For this review, take the finished solid that the model builds, in its own axes (mm). A direction names the side the tool comes from. Give positions to 0.01 mm unless a question says otherwise; leave off trailing zeros. Loops run counter-clockwise (first coordinate to the right, second up) from the corner with the lowest first, then second, coordinate; pieces in that order, holes last. Notation, with made-up numbers: (-30.75, 88) - (22.25, 88) arc R15 cw to (22.25, 116) - close; hole circle Ø2 at (83, -16). An arc over 180 degrees is marked (long way). Put each result on its own line as item: value.
Autodesk Inventor part; units mm, degrees
ref_plane "YZ Plane" through (0, 0, 0) normal (1, 0, 0) x (0, 1, 0)
ref_plane "XZ Plane" through (0, 0, 0) normal (0, 1, 0) x (-1, 0, 0)
ref_plane "XY Plane" through (0, 0, 0) normal (0, 0, 1) x (1, 0, 0)
sketch "Sketch1" plane through (0, 0, 0) normal (0, 1, 0) x (-1, 0, 0)
  line L0 (0, 0) -> (-139.7, 0)
  line L1 (-139.7, 0) -> (-139.7, -139.7)
  line L2 (-139.7, -139.7) -> (0, -139.7)
  line L3 (0, -139.7) -> (0, 0)
  dimension "d0" = 139.7
  dimension "d1" = 139.7
extrude "Extrusion1" add sketch "Sketch1" along normal blind 25.4
sketch "Sketch2" plane through (0, 25.4, 0) normal (0, 1, 0) x (1, 0, 0)
  circle A0 centre (104.775, 34.925) radius 25.4
  line L0 (0, 0) -> (139.7, 0)
  line L1 (139.7, 0) -> (139.7, 139.7)
  line L2 (139.7, 139.7) -> (0, 139.7)
  line L3 (0, 139.7) -> (0, 0)
  dimension "d4" = 50.8
  dimension "d5" = 34.925
  dimension "d6" = 34.925
extrude "Extrusion2" cut sketch "Sketch2" against normal blind 3.175 contours A0
sketch "Sketch3" plane through (104.775, 22.225, -34.925) normal (0, 1, 0) x (1, 0, 0)
  circle A0 centre (0, 0) radius 19.05
  point P0 (-104.775, -34.925)
  dimension "d9" = 38.1
extrude "Extrusion3" cut sketch "Sketch3" against normal blind 3.937
equation "\"d5\" = d6"
properties part number "Saber plaque"
1) Draft analysis for pull direction X (two halves, no side actions). For faces 1 (the face through (139.7, 13, -69)), 2 (the face through (108, 22.225, -54)), 3 (the face through (101.47, 23.83, -60.11)), 4 (the face through (71, 13, -139.7)), state which applies: pulls with the +X half, pulls with the -X half, needs draft (parallel to the pull), parting line crosses it, or undercut.
Geometry check:
face 1: pulls with the +X half
face 2: undercut
face 3: undercut
face 4: needs draft
2) Take a section at A-A on x = 98.5. State the section outline as (y, z) points (3 decimals), and give its area (3 significant figures).
Geometry check:
outline: (0, -139.7) - (25.4, -139.7) - (25.4, -59.538) - (22.225, -59.538) - (22.225, -52.912) - (18.288, -52.912) - (18.288, -16.938) - (22.225, -16.938) - (22.225, -10.312) - (25.4, -10.312) - (25.4, 0) - (0, 0) - close
area: 3,250 mm²
3) Wall thickness on line 1 (Y direction, x = 111, z = -33.5); line 2 (X direction, y = 21, z = -38); line 3 (Z direction, x = 125, y = 23.5): over which ranges is each line inside the solid? List them lowest first.
Geometry check:
line 1: y = 0 to 18.29
line 2: x = 0 to 85.97, 123.58 to 139.7
line 3: z = -139.7 to -50.29, -19.56 to 0
4) Take a section at C-C on y = 20. State the section outline as (x, z) points (3 decimals).
Geometry check:
outline: (0, -139.7) - (139.7, -139.7) - (139.7, 0) - (0, 0) - close; hole circle Ø38.1 at (104.775, -34.925)
5) Take a section at B-B on z = -31. State the section outline as (x, y) points (3 decimals).
Geometry check:
outline: (0, 0) - (139.7, 0) - (139.7, 25.4) - (129.87, 25.4) - (129.87, 22.225) - (123.416, 22.225) - (123.416, 18.288) - (86.134, 18.288) - (86.134, 22.225) - (79.68, 22.225) - (79.68, 25.4) - (0, 25.4) - close
6) For faces 5 (the face through (0, 13, -71)), 6 (the face through (105, 18.288, -35)), list the 3-axis set-ups (+Z, -Z, +X, -X, +Y, -Y) from which the entire face can be reached by the end or side of a thin tool; tool diameter is ignored.
Geometry check:
face 5: +Z, -Z, -X, +Y, -Y
face 6: +Y
7) Insertion check: pin 1 Ø19 at (x, z) = (105, -27) entering from +Y. The pin has a flat end and moves straight along its axis. Give the tip position at first contact, or say it passes through.
Geometry check:
pin 1: stops at y = 18.29
